Design review of the part built by this model. Coordinates are the model's own, in mm. A direction names the side the tool comes from. Coordinates: 2 decimals unless noted, no trailing zeros. Order: outer loops, then holes, each group sorted by start corner. A loop starts at its lowest first (then second) coordinate and runs counter-clockwise, first axis right, second up.
from build123d import *

# Parameters (mm, degrees)
SKETCH1_W           = 152.4
SKETCH1_H           = 41.275
BOSS_EXTRUDE1_DEPTH = 12.7
CUT_EXTRUDE1_DEPTH  = 7.1374


with BuildPart() as part:
    # Sketch1 → Boss-Extrude1 (new body)
    with BuildSketch(Plane.XY):
        Rectangle(SKETCH1_W, SKETCH1_H)
    extrude(amount=BOSS_EXTRUDE1_DEPTH)

    # Sketch2 → Cut-Extrude1 (cut)
    with BuildSketch(Plane.XY.offset(12.7)):
        with BuildLine():
            Line((-66.718427065, 15.875), (66.718427065, 15.875))
            ThreePointArc((66.718427065, 15.875), (70.055315538, 14.492815538), (71.4375, 11.155927065))
            Line((71.4375, 11.155927065), (71.4375, 3.131572935))
            ThreePointArc((71.4375, 3.131572935), (70.055315538, -0.205315538), (66.718427065, -1.5875))
            Line((66.718427065, -1.5875), (50.8, -1.5875))
            Line((50.8, -1.5875), (50.8, -11.155927065))
            ThreePointArc((50.8, -11.155927065), (49.417815538, -14.492815538), (46.080927065, -15.875))
            Line((46.080927065, -15.875), (-46.080927065, -15.875))
            ThreePointArc((-46.080927065, -15.875), (-49.417815538, -14.492815538), (-50.8, -11.155927065))
            Line((-50.8, -11.155927065), (-50.8, -1.5875))
            Line((-50.8, -1.5875), (-66.718427065, -1.5875))
            ThreePointArc((-66.718427065, -1.5875), (-70.055315538, -0.205315538), (-71.4375, 3.131572935))
            Line((-71.4375, 3.131572935), (-71.4375, 11.155927065))
            ThreePointArc((-71.4375, 11.155927065), (-70.055315538, 14.492815538), (-66.718427065, 15.875))
        make_face()
    extrude(amount=-CUT_EXTRUDE1_DEPTH, mode=Mode.SUBTRACT)


solid = part.part
1. Add section A-A (y = -6). Give the boundary of the cut face in (x, z).
2. For faces 1 (the flat face through (-1, -20.638, 6)), 2 (the flat face through (50.8, -6, 9)), list the 3-axis set-ups (+Z, -Z, +X, -X, +Y, -Y) from which the entire face can be reached by the end or side of a thin tool; tool diameter is ignored.
3. To check wall thickness, follow line 1 (Y direction, x = 26, z = 12) (1 decimal); line 2 (Y direction, x = -54.5, z = 8) (1 decimal); line 3 (Z direction, x = -46, y = -4). State the ranges of each line that lie inside material, in increasing order.
4. Mouldability with a two-part tool opening along X and no side actions: class faces 3 (the flat face through (76.2, 0, 6)), 4 (the flat face through (-76.2, 0, 6)), 5 (the flat face through (-6, -17, 12.7)), 6 (the flat face through (-50.8, -6, 9)) as pulls with the +X half, pulls with the -X half, needs draft (parallel to the pull), parting line crosses it, or undercut.
5. Add section B-B (z = 9). Give the boundary of the cut face in (x, y) (1 decimal).
6. Add section C-C (x = -15.5). Give the boundary of the cut face in (y, z) (1 decimal).
Solution:
1. outline: (-76.2, 0) - (76.2, 0) - (76.2, 12.7) - (50.8, 12.7) - (50.8, 5.56) - (-50.8, 5.56) - (-50.8, 12.7) - (-76.2, 12.7) - close
2. face 1: +Z, -Z, +X, -X, -Y
2. face 2: +Z
3. line 1: y = -20.6 to -15.9, 15.9 to 20.6
3. line 2: y = -20.6 to -1.6, 15.9 to 20.6
3. line 3: z = 0 to 5.56
4. face 3: pulls with the +X half
4. face 4: pulls with the -X half
4. face 5: needs draft
4. face 6: undercut
5. outline: (-76.2, -20.6) - (76.2, -20.6) - (76.2, 20.6) - (-76.2, 20.6) - close; hole (-71.4, 3.1) arc R4.7 ccw to (-66.7, -1.6) - (-50.8, -1.6) - (-50.8, -11.2) arc R4.7 ccw to (-46.1, -15.9) - (46.1, -15.9) arc R4.7 ccw to (50.8, -11.2) - (50.8, -1.6) - (66.7, -1.6) arc R4.7 ccw to (71.4, 3.1) - (71.4, 11.2) arc R4.7 ccw to (66.7, 15.9) - (-66.7, 15.9) arc R4.7 ccw to (-71.4, 11.2) - close
6. outline: (-20.6, 0) - (20.6, 0) - (20.6, 12.7) - (15.9, 12.7) - (15.9, 5.6) - (-15.9, 5.6) - (-15.9, 12.7) - (-20.6, 12.7) - close
